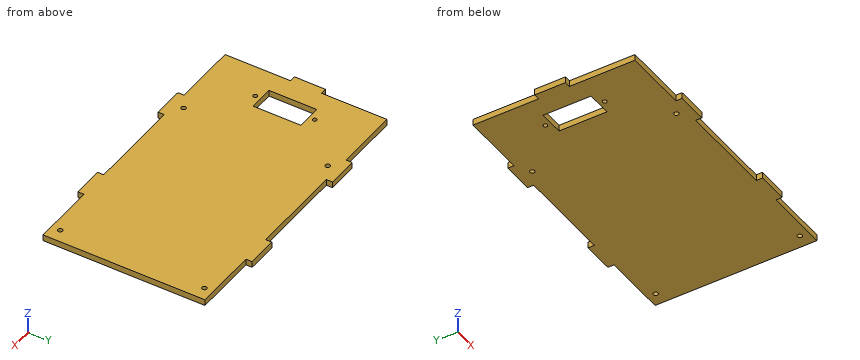
from build123d import *

# Parameters (mm, degrees)
BOSS_EXTRUDE1_DEPTH = 3
SKETCH2_R           = 1.13
CUT_EXTRUDE1_DEPTH  = 3
SKETCH3_R           = 1
SKETCH3_W           = 12.1
SKETCH3_H           = 23.2
CUT_EXTRUDE4_DEPTH  = 3


with BuildPart() as part:
    # Sketch1 → Boss-Extrude1 (new body)
    with BuildSketch(Plane.XY):
        Polygon((-36.547918648, 71.490037876), (-5.317918648, 71.490037876), (-5.317918648, 74.490037876), (9.682081352, 74.490037876), (9.682081352, 71.490037876), (55.912081352, 71.490037876), (55.912081352, 74.490037876), (70.912081352, 74.490037876), (70.912081352, 71.490037876), (102.145081352, 71.490037876), (102.142081352, -6.979962124), (70.912081352, -6.979962124), (70.912081352, -9.979962124), (55.912081352, -9.979962124), (55.912081352, -6.979962124), (9.682081352, -6.979962124), (9.682081352, -9.979962124), (-5.317918648, -9.979962124), (-5.317918648, -6.979962124), (-36.547918648, -6.979962124), (-36.547918648, 24.755037876), (-39.547918648, 24.755037876), (-39.547918648, 39.755037876), (-36.547918648, 39.755037876), align=None)
    extrude(amount=BOSS_EXTRUDE1_DEPTH)

    # Sketch2 → Cut-Extrude1 (cut)
    with BuildSketch(Plane.XY.offset(3)):
        with Locations((95.834916571, 67.180037876)):
            Circle(SKETCH2_R)
        with Locations((95.832246124, -2.669962124)):
            Circle(SKETCH2_R)
        with Locations((1.854916503, 67.180037876)):
            Circle(SKETCH2_R)
        with Locations((1.852246055, -2.669962124)):
            Circle(SKETCH2_R)
    extrude(amount=-CUT_EXTRUDE1_DEPTH, mode=Mode.SUBTRACT)

    # Sketch3 → Cut-Extrude4 (cut)
    with BuildSketch(Plane.XY.offset(3)):
        with Locations((-20.497918648, 46.660037876)):
            Circle(SKETCH3_R)
        with Locations((-20.497918648, 17.860037876)):
            Circle(SKETCH3_R)
        with Locations((-20.497918648, 32.260037876)):
            Rectangle(SKETCH3_W, SKETCH3_H)
    extrude(amount=-CUT_EXTRUDE4_DEPTH, mode=Mode.SUBTRACT)


solid = part.part
Could you check a few things on this model? Use its own coordinates, in mm. Coordinates: 2 decimals unless noted, no trailing zeros. Loops run counter-clockwise (first coordinate to the right, second up) from the corner with the lowest first, then second, coordinate; pieces in that order, holes last. Notation, with made-up numbers: (-9.75, -27) -> (31.25, -27) arc R19 ccw to (31.25, -16) -> close; hole circle Ø3 at (3.25, 0.25). An arc over 180 degrees is marked (long way). Answer in a Markdown table with one row per item.
(1) If I drill on probe 1 along X at (y, z) = (39, 1.85); probe 2 along X at (y, z) = (42, 0.35); probe 3 along Y at (x, z) = (48.5, 1.5), over which ranges is the centre line in solid material (lowest first)?
Results found:
| item | result |
|---|---|
| probe 1 | x = -39.55 to -26.55, -14.45 to 102.14 |
| probe 2 | x = -36.55 to -26.55, -14.45 to 102.14 |
| probe 3 | y = -6.98 to 71.49 |
(2) Imagine slicing it at B-B (y = 42). List the corners of the cut face in (x, z) for me.
Results found:
| item | result |
|---|---|
| outline | (-36.55, 0) -> (-26.55, 0) -> (-26.55, 3) -> (-36.55, 3) -> close; (-14.45, 0) -> (102.14, 0) -> (102.14, 3) -> (-14.45, 3) -> close |
(3) Imagine slicing it at A-A (z = 1.75). Give the number of separate pieces and of enclosed holes in the cut face, plus the area to 3 significant figures.
Results found:
| item | result |
|---|---|
| separate pieces | 1 |
| enclosed holes | 7 |
| area | 10,800 mm^2 |
(4) Imagine slicing it at C-C (x = 79.5). List the corners of the cut face in (y, z) for me, plus the area to 3 significant figures.
Results found:
| item | result |
|---|---|
| outline | (-6.98, 0) -> (71.49, 0) -> (71.49, 3) -> (-6.98, 3) -> close |
| area | 235 mm^2 |
(5) Imagine slicing it at D-D (y = 2). List the corners of the cut face in (x, z) for me.
Results found:
| item | result |
|---|---|
| outline | (-36.55, 0) -> (102.14, 0) -> (102.14, 3) -> (-36.55, 3) -> close |
(6) Will these pins go through, and if not, where does the flat tip stop? pin 1 Ø1.5 at (y, z) = (72.5, 1.5) entering from -X; pin 2 Ø1.5 at (x, z) = (-18, 1.5) entering from +Y; pin 3 Ø0.9 at (y, z) = (73.5, 1) entering from +X.
Results found:
| item | result |
|---|---|
| pin 1 | stops at x = -5.32 |
| pin 2 | stops at y = 71.49 |
| pin 3 | stops at x = 70.91 |
